Answer from the drawing. Dimensions are ordinates in mm from the lowest x, y and z of the part. Give positions to 0.01 mm unless a question says otherwise; leave off trailing zeros. Order: outer loops, then holes, each group sorted by start corner. A loop starts at its lowest first (then second) coordinate and runs counter-clockwise, first axis right, second up.
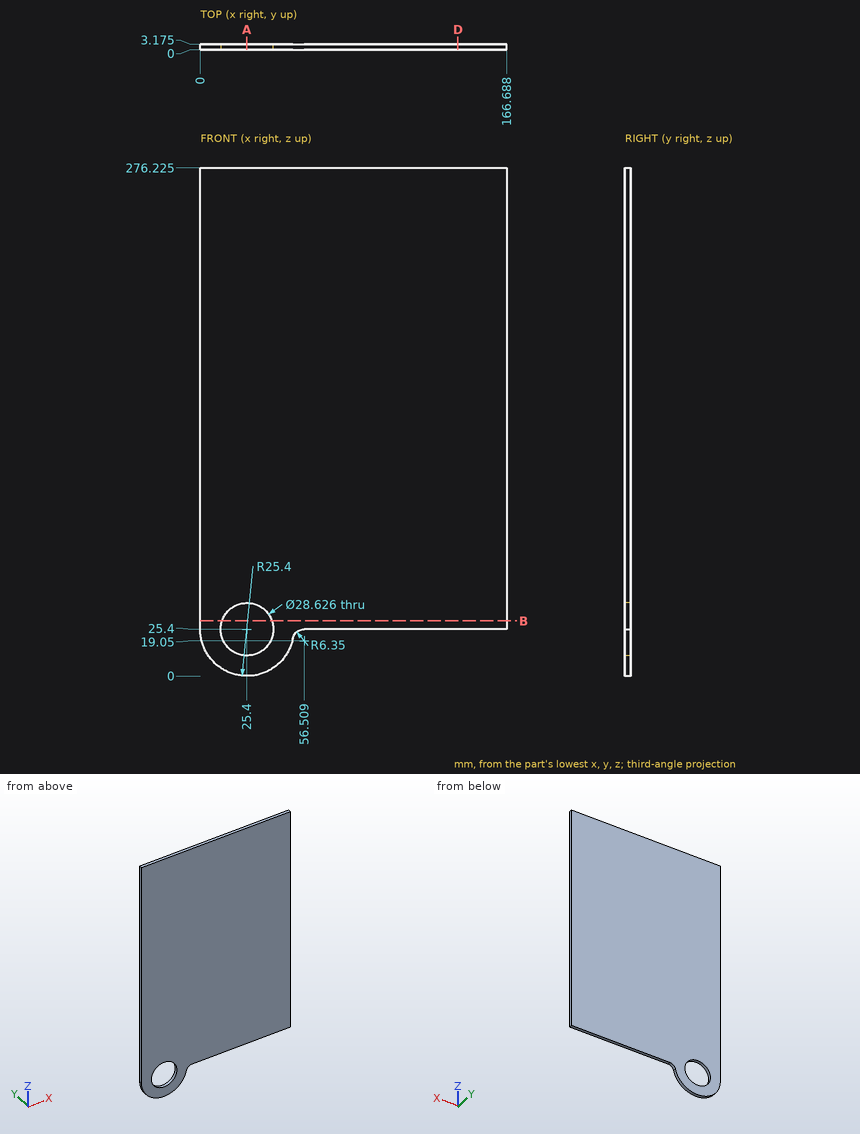
1. The part is cut by section A-A (x = 25.4). Write down the section's boundary in (y, z) (1 decimal).
Findings below:
outline: (0, 0) - (3.2, 0) - (3.2, 11.1) - (0, 11.1) - close; (0, 39.7) - (3.2, 39.7) - (3.2, 276.2) - (0, 276.2) - close
2. The part is cut by section D-D (x = 140). Write down the section's boundary in (y, z) (1 decimal).
Findings below:
outline: (0, 25.4) - (3.2, 25.4) - (3.2, 276.2) - (0, 276.2) - close
3. Straight lines are drawn through the part: probe 1 along Z at (x, y) = (25.4, 1) (1 decimal); probe 2 along Z at (x, y) = (64, 2.15) (1 decimal); probe 3 along X at (y, z) = (0.75, 26.5). For each, find the intervals that lie inside material, in ascending order.
Findings below:
probe 1: z = 0 to 11.1, 39.7 to 276.2
probe 2: z = 25.4 to 276.2
probe 3: x = 0 to 11.13, 39.67 to 166.69
4. The part is cut by section B-B (z = 30). Write down the section's boundary in (x, y) (1 decimal).
Findings below:
outline: (0, 0) - (11.8, 0) - (11.8, 3.2) - (0, 3.2) - close; (39, 0) - (166.7, 0) - (166.7, 3.2) - (39, 3.2) - close
